```python
from build123d import *

# Parameters (mm, degrees)
SKETCH1_R           = 1.5875
BOSS_EXTRUDE1_DEPTH = 1.5875


with BuildPart() as part:
    # Sketch1 → Boss-Extrude1 (new body)
    with BuildSketch(Plane(origin=(0, 0, 0), x_dir=(1, 0, 0), z_dir=(0, 1, 0))):
        with BuildLine():
            Line((96.867912936, 16.100919196), (90.894787936, 16.100919196))
            ThreePointArc((90.894787936, 16.100919196), (90.052888924, 15.752193207), (89.704162936, 14.910294196))
            Line((89.704162936, 14.910294196), (89.704162936, 8.798419196))
            ThreePointArc((89.704162936, 8.798419196), (89.355436947, 7.956520185), (88.513537936, 7.607794196))
            Line((88.513537936, 7.607794196), (86.807287936, 7.607794196))
            ThreePointArc((86.807287936, 7.607794196), (85.965388924, 7.956520185), (85.616662936, 8.798419196))
            Line((85.616662936, 8.798419196), (85.616662936, 14.910294196))
            ThreePointArc((85.616662936, 14.910294196), (85.267936947, 15.752193207), (84.426037936, 16.100919196))
            Line((84.426037936, 16.100919196), (74.325412936, 16.100919196))
            ThreePointArc((74.325412936, 16.100919196), (73.483513924, 16.449645185), (73.134787936, 17.291544196))
            Line((73.134787936, 17.291544196), (73.134787936, 34.868344196))
            ThreePointArc((73.134787936, 34.868344196), (73.483513924, 35.710243207), (74.325412936, 36.058969196))
            Line((74.325412936, 36.058969196), (89.210056936, 36.058969196))
            ThreePointArc((89.210056936, 36.058969196), (90.051955947, 36.407695185), (90.400681936, 37.249594196))
            Line((90.400681936, 37.249594196), (90.400681936, 43.684176196))
            ThreePointArc((90.400681936, 43.684176196), (90.051955947, 44.526075207), (89.210056936, 44.874801196))
            Line((89.210056936, 44.874801196), (84.055412936, 44.874801196))
            ThreePointArc((84.055412936, 44.874801196), (83.213513924, 45.223527185), (82.864787936, 46.065426196))
            Line((82.864787936, 46.065426196), (82.864787936, 55.065426196))
            ThreePointArc((82.864787936, 55.065426196), (83.213513924, 55.907325207), (84.055412936, 56.256051196))
            Line((84.055412936, 56.256051196), (96.867912936, 56.256051196))
            Line((96.867912936, 56.256051196), (96.867912936, 66.140544196))
            Line((96.867912936, 66.140544196), (9.428412936, 66.140544196))
            Line((9.428412936, 66.140544196), (9.428412936, 35.829099196))
            Line((9.428412936, 35.829099196), (16.226102936, 35.829099196))
            ThreePointArc((16.226102936, 35.829099196), (17.068001947, 35.480373207), (17.416727936, 34.638474196))
            Line((17.416727936, 34.638474196), (17.416727936, 28.138474196))
            ThreePointArc((17.416727936, 28.138474196), (17.068001947, 27.296575185), (16.226102936, 26.947849196))
            Line((16.226102936, 26.947849196), (9.428412936, 26.947849196))
            Line((9.428412936, 26.947849196), (9.428412936, 24.375238196))
            Line((9.428412936, 24.375238196), (13.802302936, 24.375238196))
            ThreePointArc((13.802302936, 24.375238196), (14.644201947, 24.026512207), (14.992927936, 23.184613196))
            Line((14.992927936, 23.184613196), (14.992927936, 16.081488196))
            ThreePointArc((14.992927936, 16.081488196), (14.644201947, 15.239589185), (13.802302936, 14.890863196))
            Line((13.802302936, 14.890863196), (9.428412936, 14.890863196))
            Line((9.428412936, 14.890863196), (9.428412936, 3.240544196))
            Line((9.428412936, 3.240544196), (96.867912936, 3.240544196))
            Line((96.867912936, 3.240544196), (96.867912936, 16.100919196))
        make_face()
        with Locations((92.613412936, 58.820544196)):
            Circle(SKETCH1_R, mode=Mode.SUBTRACT)
        with Locations((12.603412936, 10.560544196)):
            Circle(SKETCH1_R, mode=Mode.SUBTRACT)
        with Locations((92.613412936, 10.560544196)):
            Circle(SKETCH1_R, mode=Mode.SUBTRACT)
        with Locations((12.603412936, 58.820544196)):
            Circle(SKETCH1_R, mode=Mode.SUBTRACT)
        with BuildLine():
            Line((78.881537936, 49.918794196), (72.055287936, 49.918794196))
            ThreePointArc((72.055287936, 49.918794196), (71.213388924, 50.267520185), (70.864662936, 51.109419196))
            Line((70.864662936, 51.109419196), (70.864662936, 52.815669196))
            ThreePointArc((70.864662936, 52.815669196), (71.213388924, 53.657568207), (72.055287936, 54.006294196))
            Line((72.055287936, 54.006294196), (78.881537936, 54.006294196))
            ThreePointArc((78.881537936, 54.006294196), (79.723436947, 53.657568207), (80.072162936, 52.815669196))
            Line((80.072162936, 52.815669196), (80.072162936, 51.109419196))
            ThreePointArc((80.072162936, 51.109419196), (79.723436947, 50.267520185), (78.881537936, 49.918794196))
        make_face(mode=Mode.SUBTRACT)
    extrude(amount=BOSS_EXTRUDE1_DEPTH)


solid = part.part
```
The listing builds one solid part. Answer for the finished solid, in the listing's coordinates (mm). Coordinates: 2 decimals unless noted, no trailing zeros. Loops run counter-clockwise (first coordinate to the right, second up) from the corner with the lowest first, then second, coordinate; pieces in that order, holes last. Notation, with made-up numbers: M 37.5,29 L 91.5,29 A14 cw 91.5,56 Z; hole C -1.5,26.25 d10. An arc over 180 degrees is marked long. Answer as a JSON object with one key per item and string values. Group by question number.
Item 1: Each of these flat-tipped pins is pushed along its axis until it touches: P1, Ø3.5, axis at x = 12.6, z = -58.82, coming from the +Y side; P2, Ø0.8, axis at y = 1, z = -32, coming from the -X side; P3, Ø0.5, axis at y = 0.5, z = -22.5, coming from the +X side; P4, Ø0.8, axis at y = 0.5, z = -20, coming from the -X side. Where does it stop, or does it pass through?
Item 2: Consider L1, parallel to X at y = 1.3, z = -10; L2, parallel to Z at x = 75, y = 0.8; L3, parallel to X at y = 1.45, z = -12. Determine where each line is inside the solid, lowest interval first.
Item 3: Section B-B (y = 1.2) is taken. Give the number of separate pieces and of enclosed holes in the cut face, and give its area (3 significant figures).
Item 4: Section C-C (z = -47) is taken. Write down the section's boundary in (x, y).
Item 5: Determine the mould class of faces 1 (the face through (53, 1.588, -35)), 2 (the face through (14.118, 0.783, -11.037)) for opening direction Z: +Z half, -Z half, draft (parallel to the pull), parting line (faces both ways), or undercut.
Item 6: Section A-A (z = -40.5) is taken. Write down the section's boundary in (x, y).
Solved:
{
 "1": {"P1": "stops at y = 1.59", "P2": "stops at x = 17.42", "P3": "stops at x = 73.13", "P4": "stops at x = 14.99"},
 "2": {"L1": "x = 9.43 to 11.12, 14.09 to 85.62, 89.7 to 91.13, 94.1 to 96.87", "L2": "z = -66.14 to -54.01, -49.92 to -36.06, -16.1 to -3.24", "L3": "x = 9.43 to 11.93, 13.27 to 85.62, 89.7 to 91.94, 93.28 to 96.87"},
 "3": {"separate pieces": "1", "enclosed holes": "5", "area": "4,590 mm2"},
 "4": {"outline": "M 9.43,0 L 82.86,0 L 82.86,1.59 L 9.43,1.59 Z"},
 "5": {"face 1": "draft", "face 2": "undercut"},
 "6": {"outline": "M 9.43,0 L 90.4,0 L 90.4,1.59 L 9.43,1.59 Z"}
}
